Can you work these out from the model? Positions are in its coordinate system, mm. A direction names the side the tool comes from. Round coordinates to 2 decimals unless told otherwise and drop trailing zeros. Write each loop counter-clockwise with the first axis right and the second up, starting at its lowest first coordinate (ties: lowest second). Pieces come first, ordered by that corner, then holes. Notation, with made-up numbers: M 3,75.25 L 31,75.25 A10 cw 31,87.25 Z; hole C 10,58 d10. An arc over 180 degrees is marked long. Answer as a JSON object with one key per item and string values. Group by question number.
1) Suppose I cut it at C-C, the plane y = 0. Write out the boundary of the cut face in (x, z), and give its area (3 significant figures).
2) On a 3-axis mill with a long thin cutter (end or side, diameter ignored), from which of +Z, -Z, +X, -X, +Y, -Y can I reach the whole of each face in a straight line? I mean faces 4 (the cylindrical face through (-16.153, -6.699, 6.785)), 5 (the cylindrical face through (-0.762, -10.479, 11.074)), 6 (the flat face through (-16, 11, 6.5)). Say none if no direction works.
3) If we mould it in two halves opening along Y, with no side actions, what happens to faces 1 (the cylindrical face through (-0.762, 0.084, 11.074)), 2 (the flat face through (-7.7, -12, 7.7)), 3 (the cylindrical face through (0, 7.5, 16.1))? For each: +Y half, -Y half, draft (parallel to the pull), parting line (faces both ways), or undercut.
4) Suppose I cut it at A-A, the plane x = -14. Write out the boundary of the cut face in (y, z).
5) Suppose I cut it at B-B, the plane z = 14. Write out the boundary of the cut face in (x, y).
6) Please list where these lines run through material, in increasing order: L1, parallel to Y at x = -4.5, z = 13.75; L2, parallel to Y at x = -14, z = 6.25; L3, parallel to X at y = 7.5, z = 12. Write a range as [from, to].
7) I'm going to push flat-ended pins straight in: pin 1 Ø4.5 at (x, z) = (-3, 11) entering from +Y; pin 2 Ø6 at (x, z) = (-19, 14) entering from -Y; pin 3 Ø3.5 at (x, y) = (-19, -2) entering from +Z; pin 4 Ø2 at (x, z) = (4, 13.5) entering from -Y. Where does each tip first touch, or does it pass through?
8) Suppose I cut it at D-D, the plane y = 6.5. Write out the boundary of the cut face in (x, z), and give its area (3 significant figures).
from build123d import *

# Parameters (mm, degrees)
BOSS_EXTRU_1_DEPTH      = 12
BOSS_EXTRU_2_START      = -4
BOSS_EXTRU_2_DEPTH      = 1
CONG_1_R                = 1
ESQUISSE3_R             = 1.5
ENL_V_MAT_EXTRU_1_DEPTH = 28.66152567


with BuildPart() as part:
    # Esquisse1 → Boss.-Extru.1 (new, symmetric)
    with BuildSketch(Plane(origin=(0, 0, 0), x_dir=(1, 0, 0), z_dir=(0, 1, 0))):
        with BuildLine():
            Line((7.5, -6.76461381), (7.5, -8.182909018))
            ThreePointArc((7.5, -8.182909018), (-1.126445761, -11.042695321), (-8.997777503, -6.5))
            Line((-8.997777503, -6.5), (-23, -6.5))
            Line((-23, -6.5), (-23, -5.5))
            Line((-23, -5.5), (-8, -5.5))
            Line((-8, -5.5), (-8, -6.165225057))
            ThreePointArc((-8, -6.165225057), (-0.390277747, -10.092456751), (7.5, -6.76461381))
        make_face()
    extrude(amount=BOSS_EXTRU_1_DEPTH, both=True)

    # Esquisse2 → Boss.-Extru.2 (add)
    with BuildSketch(Plane(origin=(0, 12, 0), x_dir=(1, 0, 0), z_dir=(0, 1, 0)).offset(BOSS_EXTRU_2_START)):
        with BuildLine():
            Line((7.5, -8.182909018), (7.5, -14.246403055))
            ThreePointArc((7.5, -14.246403055), (0.168377113, -16.099119515), (-7.200392055, -14.400151188))
            Line((-7.200392055, -14.400151188), (-23, -6.5))
            Line((-23, -6.5), (-8.997777503, -6.5))
            ThreePointArc((-8.997777503, -6.5), (-1.126445761, -11.042695321), (7.5, -8.182909018))
        make_face()
    boss_extru_2 = extrude(amount=-BOSS_EXTRU_2_DEPTH)

    # Symétrie1: Boss.-Extru.2 across plane
    add(boss_extru_2.mirror(Plane.ZX))

    # Congé1
    cong_1_edges = [part.edges().sort_by_distance(p)[0] for p in [
        (-8.997777503, 10, 6.5),
        (7.5, 12, 7.473761414),
        (-8.997777503, 0, 6.5),
        (-1.126445761, 7, 11.042695321),
        (7.5, 7.5, 14.246403055),
        (-15.998888752, 7, 6.5),
        (-1.126445761, 8, 11.042695321),
        (-15.998888752, 8, 6.5),
        (-8.997777503, -10, 6.5),
        (-23, 12, 6),
        (-1.126445761, -8, 11.042695321),
        (-15.998888752, -8, 6.5),
        (7.5, -7.5, 14.246403055),
        (-1.126445761, -7, 11.042695321),
        (-15.998888752, -7, 6.5),
        (7.5, -12, 7.473761414),
        (-23, -12, 6),
    ]]
    fillet(cong_1_edges, radius=CONG_1_R)

    # Esquisse3 → Enlèv. mat.-Extru.1 (cut, through all)
    with BuildSketch(Plane.XY.offset(6.5)):
        with Locations((-14, 0)):
            Circle(ESQUISSE3_R)
    extrude(amount=-ENL_V_MAT_EXTRU_1_DEPTH, mode=Mode.SUBTRACT)


solid = part.part
Results:
{
 "1": {"outline": "M -23,5.5 L -15.5,5.5 L -15.5,6.5 L -23,6.5 Z; M -12.5,5.5 L -8,5.5 L -8,6.17 A10.1 cw 7.5,6.76 L 7.5,8.18 A11.1 ccw -8.71,6.88 A1 cw -9.5,6.5 L -12.5,6.5 Z", "area": "30.1 mm^2"},
 "2": {"face 4": "+Z, -X", "face 5": "+Z, -Y", "face 6": "+Z, -X, +Y"},
 "3": {"face 1": "undercut", "face 2": "-Y half", "face 3": "draft"},
 "4": {"outline": "M -12,5.5 L -1.5,5.5 L -1.5,6.5 L -6,6.5 A1 cw -7,7.5 L -7,11 L -8,11 L -8,7.5 A1 cw -9,6.5 L -12,6.5 Z; M 1.5,5.5 L 12,5.5 L 12,6.5 L 9,6.5 A1 cw 8,7.5 L 8,11 L 7,11 L 7,7.5 A1 cw 6,6.5 L 1.5,6.5 Z"},
 "5": {"outline": "M -8,-8 L 7.43,-8 L 7.43,-7 L -8,-7 Z; M -8,7 L 7.43,7 L 7.43,8 L -8,8 Z"},
 "6": {"L1": "[-8, -7], [7, 8]", "L2": "[-12, -1.5], [1.5, 12]", "L3": "[-12, 7.5]"},
 "7": {"pin 1": "y = 12", "pin 2": "through", "pin 3": "z = 6.5", "pin 4": "y = -8"},
 "8": {"outline": "M -23,5.5 L -8,5.5 L -8,6.17 A10.1 cw 7.5,6.76 L 7.5,8.36 A11.23 ccw -8.82,6.96 A0.87 cw -9.5,6.63 L -22.73,6.63 L -23,6.5 Z", "area": "37.4 mm^2"}
}
